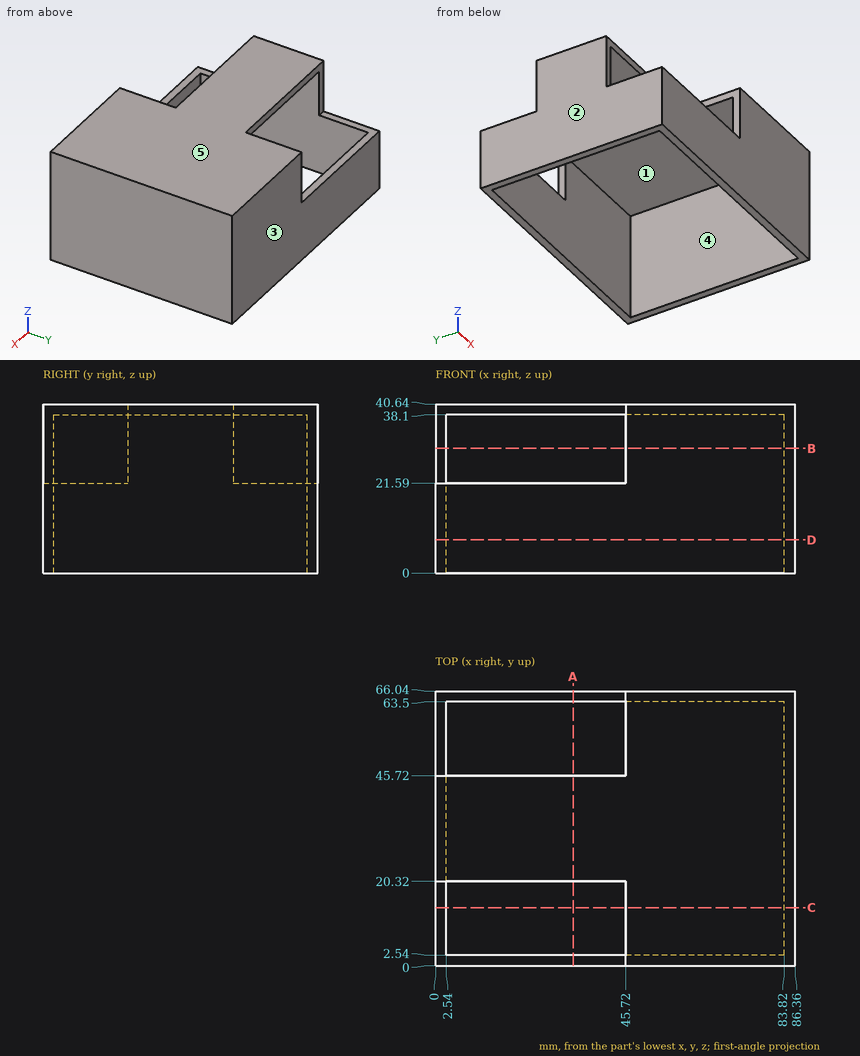
Source: three-view drawing plus pictorial views. Frame: mm from the lowest corner of the part. A direction names the side the tool comes from. Round coordinates to 2 decimals unless told otherwise and drop trailing zeros. Loops run counter-clockwise (first coordinate to the right, second up) from the corner with the lowest first, then second, coordinate; pieces in that order, holes last.
1. Section query B-B on z = 30. Output: boundary loops of the cut face in (x, y), and give its area (3 significant figures).
2. Mould query, pull axis X, two halves, no side actions, for the marked faces 1, 2 and 3. Classes: released by +X, released by -X, zero draft, split by the parting line, or undercut.
3. Ray query, L1, parallel to Y at x = 80, z = 2.5; L2, parallel to X at y = 54, z = 13; L3, parallel to Z at x = 52.5, y = 21. Return the intervals inside material, ascending.
4. Section query A-A on x = 33. Output: boundary loops of the cut face in (y, z).
5. Section query C-C on y = 14. Output: boundary loops of the cut face in (x, z).
6. Access query for the marked faces 4 and 5. Directions: +Z, -Z, +X, -X, +Y, -Y. A direction counts if a zero-diameter tool reaches every point of the face in a straight line with its end or side. Return the directions, or none.
7. Section query D-D on z = 8. Output: boundary loops of the cut face in (x, y).
8. Contact query for flat-ended pins moving along their axis: pin 1 (1.5 mm diameter, centred on x = 26.5, y = 46, fed in from -Z); pin 2 (16.5 mm diameter, centred on x = 16.5, y = 6, fed in from +Z); pin 3 (9.5 mm diameter, centred on y = 60, z = 30.5, fed in from -X). Output: stop coordinate, or through.
Answers below:
1. outline: (0, 20.32) - (2.54, 20.32) - (2.54, 45.72) - (0, 45.72) - close; (45.72, 0) - (86.36, 0) - (86.36, 66.04) - (45.72, 66.04) - (45.72, 63.5) - (83.82, 63.5) - (83.82, 2.54) - (45.72, 2.54) - close
1. area: 426 mm2
2. face 1: undercut
2. face 2: released by -X
2. face 3: zero draft
3. L1: y = 0 to 2.54, 63.5 to 66.04
3. L2: x = 0 to 2.54, 83.82 to 86.36
3. L3: z = 38.1 to 40.64
4. outline: (0, 0) - (2.54, 0) - (2.54, 21.59) - (0, 21.59) - close; (20.32, 38.1) - (45.72, 38.1) - (45.72, 40.64) - (20.32, 40.64) - close; (63.5, 0) - (66.04, 0) - (66.04, 21.59) - (63.5, 21.59) - close
5. outline: (0, 0) - (2.54, 0) - (2.54, 21.59) - (0, 21.59) - close; (45.72, 38.1) - (83.82, 38.1) - (83.82, 0) - (86.36, 0) - (86.36, 40.64) - (45.72, 40.64) - close
6. face 4: -Z
6. face 5: +Z, +X, -X, +Y, -Y
7. outline: (0, 0) - (86.36, 0) - (86.36, 66.04) - (0, 66.04) - close; hole (2.54, 2.54) - (83.82, 2.54) - (83.82, 63.5) - (2.54, 63.5) - close
8. pin 1: stops at z = 38.1
8. pin 2: stops at z = 21.59
8. pin 3: stops at x = 45.72
